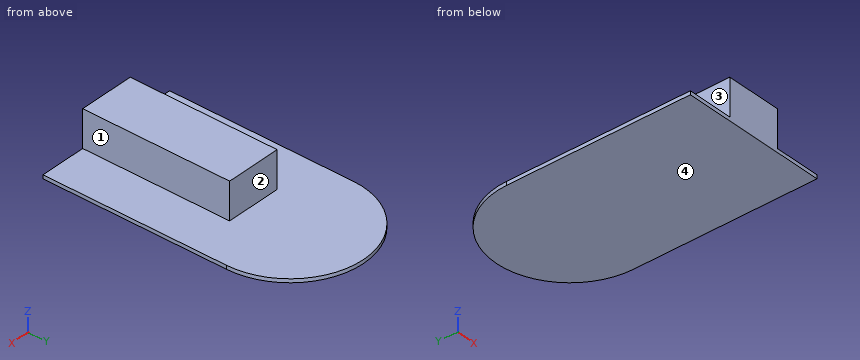
```python
from build123d import *

# Parameters (mm, degrees)
F0_W     = 40
F0_H     = 50
F1_DEPTH = 1
F2_W     = 15
F2_H     = 40
F3_DEPTH = 10


with BuildPart() as f1:
    # F0 (on Top) → F1 (new body)
    with BuildSketch(Plane.XY):
        with Locations((-114.646277, 15.575861)):
            Rectangle(F0_W, F0_H)
        with BuildLine():
            ThreePointArc((-94.646277, 40.575861), (-114.646277, 60.575861), (-134.646277, 40.575861))
            Line((-134.646277, 40.575861), (-94.646277, 40.575861))
        make_face()
    extrude(amount=F1_DEPTH)

    # F2 (on face) → F3 (join)
    with BuildSketch(Plane.XY.offset(1)):
        with Locations((-114.680499, 10.575861)):
            Rectangle(F2_W, F2_H)
    extrude(amount=F3_DEPTH)


solid = f1.part
```
The model under review builds one solid part; all positions refer to its coordinate system, in mm. Face numbers are marked on the shaded views. A direction names the side the tool comes from. Round coordinates to 2 decimals unless told otherwise and drop trailing zeros. Write each loop counter-clockwise with the first axis right and the second up, starting at its lowest first coordinate (ties: lowest second). Pieces come first, ordered by that corner, then holes.
(1) We need section C-C on x = -110. Give the boundary of the cut face in (y, z).
(2) Insertion check: pin 1 (5 mm diameter, centred on y = 12, z = 4, fed in from +X); pin 2 (5 mm diameter, centred on y = 4, z = 6.5, fed in from -X). Each pin has a flat end and moves straight along its axis. Give the tip position at first contact, or say it passes through.
(3) We need section D-D on x = -119.5. Give the boundary of the cut face in (y, z), and give its area (3 significant figures).
(4) We need section A-A on y = 17. Give the boundary of the cut face in (x, z), and give its area (3 significant figures).
(5) Machinability: for the marked faces 1, 2, 3 and 4, which of the approach directions +Z, -Z, +X, -X, +Y, -Y give a long, thin tool a straight path to every point of the face, cutting with its end or side? Answer none if there is none.
(6) We need section B-B on z = 8.75. Give the boundary of the cut face in (x, y), and give its area (3 significant figures).
(7) Wall thickness on L1, parallel to Z at x = -131, y = 32; L2, parallel to Y at x = -111, z = 5.5; L3, parallel to X at y = 16.5, z = 6: over which ranges is each line inside the solid? List them lowest first.
Findings below:
1. outline: (-9.42, 0) - (60.03, 0) - (60.03, 1) - (30.58, 1) - (30.58, 11) - (-9.42, 11) - close
2. pin 1: stops at x = -107.18
2. pin 2: stops at x = -122.18
3. outline: (-9.42, 0) - (59.98, 0) - (59.98, 1) - (30.58, 1) - (30.58, 11) - (-9.42, 11) - close
3. area: 469 mm2
4. outline: (-134.65, 0) - (-94.65, 0) - (-94.65, 1) - (-107.18, 1) - (-107.18, 11) - (-122.18, 11) - (-122.18, 1) - (-134.65, 1) - close
4. area: 190 mm2
5. face 1: +Z, +X, +Y, -Y
5. face 2: +Z, +X, -X, +Y
5. face 3: +Z, -X, +Y, -Y
5. face 4: -Z, +X, -X, +Y, -Y
6. outline: (-122.18, -9.42) - (-107.18, -9.42) - (-107.18, 30.58) - (-122.18, 30.58) - close
6. area: 600 mm2
7. L1: z = 0 to 1
7. L2: y = -9.42 to 30.58
7. L3: x = -122.18 to -107.18
